from build123d import *

# Parameters (mm, degrees)
SKETCH1_W           = 130
SKETCH1_H           = 210
BOSS_EXTRUDE1_DEPTH = 10
SKETCH2_W           = 130
SKETCH2_H           = 210
SKETCH2_W_2         = 120
SKETCH2_H_2         = 200
BOSS_EXTRUDE2_DEPTH = 30
BOSS_EXTRUDE3_DEPTH = 3


with BuildPart() as part:
    # Sketch1 → Boss-Extrude1 (new body)
    with BuildSketch(Plane(origin=(0, 0, 0), x_dir=(1, 0, 0), z_dir=(0, 1, 0))):
        with Locations((65, 105)):
            Rectangle(SKETCH1_W, SKETCH1_H)
    extrude(amount=BOSS_EXTRUDE1_DEPTH)

    # Sketch2 → Boss-Extrude2 (add)
    with BuildSketch(Plane(origin=(0, 10, 0), x_dir=(1, 0, 0), z_dir=(0, 1, 0))):
        with Locations((65, 105)):
            Rectangle(SKETCH2_W, SKETCH2_H)
        with Locations((65, 105)):
            Rectangle(SKETCH2_W_2, SKETCH2_H_2, mode=Mode.SUBTRACT)
    extrude(amount=BOSS_EXTRUDE2_DEPTH)

    # Sketch3 → Boss-Extrude3 (add)
    # profile 1 of 3: a face of its own
    with BuildSketch(Plane.XY):
        Polygon((53.333333333, 30), (58.717948718, 30), (58.717948718, 28.205128205), (56.923076923, 28.205128205), (56.923076923, 20), (55.128205128, 20), (55.128205128, 28.205128205), (53.333333333, 28.205128205), align=None)
    # profile 2 of 3: a face of its own
    with BuildSketch(Plane.XY):
        Polygon((60.128205128, 30), (65.512820513, 30), (65.512820513, 28.205128205), (61.923076923, 28.205128205), (61.923076923, 26.282051282), (65.512820513, 26.282051282), (65.512820513, 24.487179487), (61.923076923, 24.487179487), (61.923076923, 21.794871795), (65.512820513, 21.794871795), (65.512820513, 20), (60.128205128, 20), align=None)
    # profile 3 of 3: a face of its own
    with BuildSketch(Plane.XY):
        Polygon((70.38661859, 30), (72.051282051, 30), (76.08974359, 20), (74.172676282, 20), (73.395432692, 22.051282051), (69.038461538, 22.051282051), (68.261217949, 20), (66.346153846, 20), align=None)
        Polygon((71.217948718, 27.317708333), (69.719551282, 23.846153846), (72.716346154, 23.846153846), align=None, mode=Mode.SUBTRACT)
    extrude(amount=BOSS_EXTRUDE3_DEPTH)


solid = part.part
Input: part model. Units: mm. Frame: model coordinates. A direction names the side the tool comes from. Coordinates: 2 decimals unless noted, no trailing zeros. Loops run counter-clockwise (first coordinate to the right, second up) from the corner with the lowest first, then second, coordinate; pieces in that order, holes last.
Q1. Cut plane B-B (z = -113). Output: boundary loops of the cut face in (x, y).
Q2. Cut plane A-A (y = 13). Output: boundary loops of the cut face in (x, z).
Q3. Set-up query: faces 4 (the face through (64, 25, -5)), 5 (the face through (74.042, 25.07, 1.479)), 6 (the face through (68.34, 24.93, 1.48)). Return all of +Z, -Z, +X, -X, +Y, -Y with unobstructed straight access to the full face (end or side cutting, diameter ignored); none if empty.
Q4. Material intervals for line 1 (Z direction, x = 112, y = 19.5); line 2 (X direction, y = 38, z = -26); line 3 (Y direction, x = 37, z = -198.5), sorted ascending.
Q5. Cut plane C-C (x = 102.5). Output: boundary loops of the cut face in (y, z), then the cut area to 3 significant figures.
Q6. Draft query along X for faces 1 (the face through (64, 10, -106)), 2 (the face through (130, 20, -104)), 3 (the face through (70, 25, 3)). Return one class per face: +X half, -X half, draft (parallel to the pull), parting line (faces both ways), or undercut.
Q7. Contact query for flat-ended pins moving along their axis: pin 1 (1.4 mm diameter, centred on y = 29.5, z = 1, fed in from -X); pin 2 (0.9 mm diameter, centred on x = 63.5, z = 1.5, fed in from +Y); pin 3 (6 mm diameter, centred on y = 6, z = -121, fed in from -X); pin 4 (0.5 mm diameter, centred on y = 29, z = 2, fed in from +X). Output: stop coordinate, or through.
Working result:
1. outline: (0, 0) - (130, 0) - (130, 40) - (125, 40) - (125, 10) - (5, 10) - (5, 40) - (0, 40) - close
2. outline: (0, -210) - (130, -210) - (130, 0) - (0, 0) - close; hole (5, -205) - (125, -205) - (125, -5) - (5, -5) - close
3. face 4: +Y
3. face 5: +Z, +X, +Y
3. face 6: +Z, +Y
4. line 1: z = -210 to -205, -5 to 0
4. line 2: x = 0 to 5, 125 to 130
4. line 3: y = 0 to 10
5. outline: (0, -210) - (40, -210) - (40, -205) - (10, -205) - (10, -5) - (40, -5) - (40, 0) - (0, 0) - close
5. area: 2,400 mm2
6. face 1: undercut
6. face 2: +X half
6. face 3: draft
7. pin 1: stops at x = 53.33
7. pin 2: stops at y = 30
7. pin 3: stops at x = 0
7. pin 4: stops at x = 72.56
